Part model, mm, in its own coordinate system. Face numbers are marked on the shaded views. Round coordinates to 2 decimals unless told otherwise and drop trailing zeros. Loops run counter-clockwise (first coordinate to the right, second up) from the corner with the lowest first, then second, coordinate; pieces in that order, holes last.
(1) Cut at B-B on y = 22.25. Count the separate pieces of the cut face and the enclosed holes in it, then the cut area to 3 significant figures.
(2) Mould opens along Z. For the marked faces 1, 2 and 3 say: +Z half, -Z half, draft (parallel to the pull), parting line (faces both ways), or undercut.
(3) Flat gauge pins, fed straight in: pin 1 (4.5 mm diameter, centred on x = 30, z = 0, fed in from -Y); pin 2 (1 mm diameter, centred on x = -12, y = 19.5, fed in from -Z); pin 3 (6 mm diameter, centred on x = -21.21, z = 21.21, fed in from -Y). Where does each tip first touch, or does it go through?
(4) Probe probe 1 along Z at (x, y) = (0, 23.5); probe 2 along X at (y, z) = (26.25, -19.5); probe 3 along Y at (x, z) = (18.5, -21.5). List the from-to ranges inside material, lowest first.
(5) Cut at A-A on y = 11.25. List the corners of the cut face in (x, z).
from build123d import *

# Parameters (mm, degrees)
SKETCH_1_R             = 45
EXTRUDE_1_DEPTH        = 30
SKETCH_2_R             = 43
CUT_EXTRUDE_1_DEPTH    = 15
CUT_EXTRUDE_2_DEPTH    = 20
FILLET_1_R             = 5
HOLE_WIZARD_M6_1_D     = 5
HOLE_WIZARD_M6_1_DEPTH = 13
HOLE_WIZARD_M6_1_TIP   = 1.502151548
HOLE_WIZARD_M4_1_D     = 3.3
HOLE_WIZARD_M4_1_DEPTH = 8
HOLE_WIZARD_M4_1_TIP   = 0.991420021


with BuildPart() as part:
    # 草圖1 → 填料-伸長1 (new body)
    with BuildSketch(Plane(origin=(0, 0, 0), x_dir=(1, 0, 0), z_dir=(0, 1, 0))):
        with Locations(Location((0, 0, 0), (0, 0, 270))):
            Circle(SKETCH_1_R)
    extrude(amount=EXTRUDE_1_DEPTH)

    # 草圖2 → 除料-伸長1 (cut)
    with BuildSketch(Plane(origin=(0, 0, 0), x_dir=(-1, 0, 0), z_dir=(0, -1, 0))):
        with Locations(Location((0, 0, 0), (0, 0, 90))):
            Circle(SKETCH_2_R)
    extrude(amount=-CUT_EXTRUDE_1_DEPTH, mode=Mode.SUBTRACT)

    # 草圖3 → 除料-伸長2 (cut)
    with BuildSketch(Plane.XZ):
        Polygon((-47.5, 10), (-10, 10), (-10, 47.5), (10, 47.5), (10, 10), (47.5, 10), (47.5, -10), (10, -10), (10, -47.5), (-10, -47.5), (-10, -10), (-47.5, -10), align=None)
    extrude(amount=-CUT_EXTRUDE_2_DEPTH, mode=Mode.SUBTRACT)

    # 圓角1
    fillet_1_edges = [part.edges().sort_by_distance(p)[0] for p in [
        (0, 30, -45),
    ]]
    fillet(fillet_1_edges, radius=FILLET_1_R)

    # M6 螺紋孔1
    with Locations(Plane(origin=(0, 15, 0), x_dir=(-1, 0, 0), z_dir=(0, -1, 0))):
        with Locations((21.213203436, -21.213203436), (-21.213203436, 21.213203436), (-21.213203436, -21.213203436), (21.213203436, 21.213203436)):
            Hole(HOLE_WIZARD_M6_1_D / 2, depth=HOLE_WIZARD_M6_1_DEPTH)
            with Locations((0, 0, -(HOLE_WIZARD_M6_1_DEPTH + HOLE_WIZARD_M6_1_TIP / 2))):  # 118° drill point
                Cone(0, HOLE_WIZARD_M6_1_D / 2, HOLE_WIZARD_M6_1_TIP, mode=Mode.SUBTRACT)

    # M4 螺紋孔1
    with Locations(Plane(origin=(0, 20, 0), x_dir=(-1, 0, 0), z_dir=(0, -1, 0))):
        with Locations((0, -30), (0, 30), (30, 0), (-30, 0)):
            Hole(HOLE_WIZARD_M4_1_D / 2, depth=HOLE_WIZARD_M4_1_DEPTH)
            with Locations((0, 0, -(HOLE_WIZARD_M4_1_DEPTH + HOLE_WIZARD_M4_1_TIP / 2))):  # 118° drill point
                Cone(0, HOLE_WIZARD_M4_1_D / 2, HOLE_WIZARD_M4_1_TIP, mode=Mode.SUBTRACT)


solid = part.part
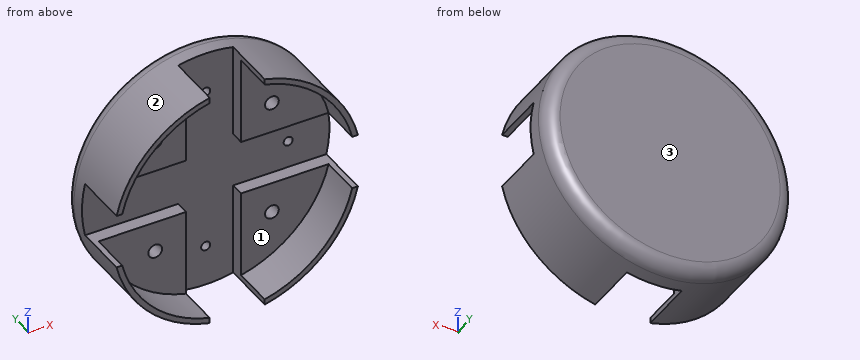
Final values:
1. separate pieces: 1
1. enclosed holes: 8
1. area: 6,250 mm2
2. face 1: undercut
2. face 2: parting line
2. face 3: draft
3. pin 1: stops at y = 20
3. pin 2: stops at z = -43.51
3. pin 3: stops at y = 15
4. probe 1: z = -45 to -31.65, -28.35 to 28.35, 31.65 to 45
4. probe 2: x = -40.38 to -23.03, -19.39 to 19.39, 23.03 to 40.38
4. probe 3: y = 15 to 30
5. outline: (-43.87, -10) arc R45 ccw to (-10, -43.87) - (-10, -41.82) arc R43 cw to (-41.82, -10) - close; (-43.87, 10) - (-41.82, 10) arc R43 cw to (-10, 41.82) - (-10, 43.87) arc R45 ccw to start; (10, -43.87) arc R45 ccw to (43.87, -10) - (41.82, -10) arc R43 cw to (10, -41.82) - close; (10, 41.82) arc R43 cw to (41.82, 10) - (43.87, 10) arc R45 ccw to (10, 43.87) - close
